```python
from build123d import *

# Parameters (mm, degrees)
SKETCH_R     = 75
PAD_DEPTH    = 200
SKETCH001_R  = 12.5
PAD001_DEPTH = 50
FILLET_R     = 20
FILLET001_R  = 20


with BuildPart() as part:
    # Sketch → Pad (new body)
    with BuildSketch(Plane.XZ):
        Circle(SKETCH_R)
    extrude(amount=PAD_DEPTH)

    # Sketch001 → Pad001 (join)
    with BuildSketch(Plane.XZ):
        Circle(SKETCH001_R)
    extrude(amount=-PAD001_DEPTH)

    # Fillet
    fillet_edges = [part.edges().sort_by_distance(p)[0] for p in [
        (-75, 0, 0),
    ]]
    fillet(fillet_edges, radius=FILLET_R)

    # Fillet001
    fillet001_edges = [part.edges().sort_by_distance(p)[0] for p in [
        (-75, -200, 0),
    ]]
    fillet(fillet001_edges, radius=FILLET001_R)


solid = part.part
```
Part model, mm, in its own coordinate system. A direction names the side the tool comes from. Coordinates: 2 decimals unless noted, no trailing zeros. Order: outer loops, then holes, each group sorted by start corner. A loop starts at its lowest first (then second) coordinate and runs counter-clockwise, first axis right, second up. Notation, with made-up numbers: (86, -7) - (137, -7) arc R23 ccw to (137, 30) - close; hole circle Ø6 at (35, -32.5). An arc over 180 degrees is marked (long way). Return JSON: item names as keys, results as strings. Group by question number.
Item 1: Cut at A-A (x = 0). List the corners of the cut face in (y, z), plus the area to 3 significant figures.
Item 2: Cut at D-D (y = 30). List the corners of the cut face in (x, z), plus the area to 3 significant figures.
Item 3: Pull direction X, two halves, no side cores. Call faces 1 (the face through (-9.764, -98.88, 74.362)), 2 (the face through (-1, -200, 1)): pulls with the +X half, pulls with the -X half, needs draft (parallel to the pull), parting line crosses it, or undercut.
Item 4: Cut at B-B (z = 0). List the corners of the cut face in (x, y), plus the area to 3 significant figures.
Item 5: Pin check, flat tips, straight feed: pin 1 (12 mm diameter, centred on y = -19.5, z = 27, fed in from -X); pin 2 (1.5 mm diameter, centred on x = -32, y = -157.5, fed in from +Z); pin 3 (4 mm diameter, centred on y = -4.5, z = 27, fed in from -X). Stop position of each tip, or through.
Item 6: Cut at C-C (y = -74.5). List the corners of the cut face in (x, z).
Item 7: Drill centre lines: probe 1 along Y at (x, z) = (-12, -6); probe 2 along Z at (x, y) = (-2, -78); probe 3 along X at (y, z) = (-138, -51). Where is each one in solid material? Low to high. Write a range as from..to.
Item 8: Which spindle directions (+Z, -Z, +X, -X, +Y, -Y) get a long thin tool onto all of the face, cutting with end or side? Do faces 3 (the face through (0, 50, 0)), 4 (the face through (11.923, 24.65, 3.755)). Say none if no direction does.
Check values:
{
 "1": {"outline": "(-200, -55) arc R20 ccw to (-180, -75) - (-20, -75) arc R20 ccw to (0, -55) - (0, -12.5) - (50, -12.5) - (50, 12.5) - (0, 12.5) - (0, 55) arc R20 ccw to (-20, 75) - (-180, 75) arc R20 ccw to (-200, 55) - close", "area": "30,900 mm2"},
 "2": {"outline": "circle Ø25 at (0, 0)", "area": "491 mm2"},
 "3": {"face 1": "parting line crosses it", "face 2": "needs draft"},
 "4": {"outline": "(-75, -180) arc R20 ccw to (-55, -200) - (55, -200) arc R20 ccw to (75, -180) - (75, -20) arc R20 ccw to (55, 0) - (12.5, 0) - (12.5, 50) - (-12.5, 50) - (-12.5, 0) - (-55, 0) arc R20 ccw to (-75, -20) - close", "area": "30,900 mm2"},
 "5": {"pin 1": "stops at x = -72", "pin 2": "stops at z = 68.18", "pin 3": "stops at x = -64.48"},
 "6": {"outline": "circle Ø150 at (0, 0)"},
 "7": {"probe 1": "y = -200..0", "probe 2": "z = -74.97..74.97", "probe 3": "x = -54.99..54.99"},
 "8": {"face 3": "+Z, -Z, +X, -X, +Y", "face 4": "+Y"}
}
